Can you work these out from the model? Positions are in its coordinate system, mm. Coordinates: 2 decimals unless noted, no trailing zeros. Loops run counter-clockwise (first coordinate to the right, second up) from the corner with the lowest first, then second, coordinate; pieces in that order, holes last.
```python
from build123d import *

# Parameters (mm, degrees)
SKICA1_W                = 30
SKICA1_H                = 160
P_IDAT_VYSUNUT_M1_DEPTH = 10
ZAOBLIT1_R              = 10


with BuildPart() as part:
    # Skica1 → Přidat vysunutím1 (new body)
    with BuildSketch(Plane.XY):
        with Locations((15, 80)):
            Rectangle(SKICA1_W, SKICA1_H)
    extrude(amount=P_IDAT_VYSUNUT_M1_DEPTH)

    # Zaoblit1
    zaoblit1_edges = [part.edges().sort_by_distance(p)[0] for p in [
        (0, 160, 5),
        (30, 160, 5),
        (30, 0, 5),
        (0, 0, 5),
    ]]
    fillet(zaoblit1_edges, radius=ZAOBLIT1_R)


solid = part.part
```
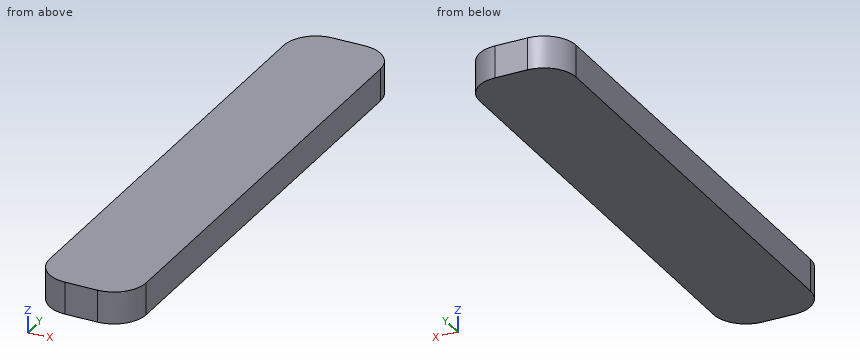
(1) I want a section at B-B on x = 2. Write out the boundary of the cut face in (y, z).
Check values:
outline: (4, 0) - (156, 0) - (156, 10) - (4, 10) - close
(2) I'm going to push a flat-ended pin straight in: pin 1 (6 mm diameter, centred on x = 26, z = 7.5, fed in from -Y). Where does the tip first touch, or does it pass through?
Check values:
pin 1: stops at y = 0.46
(3) If I drill on probe 1 along Y at (x, z) = (9.5, 9); probe 2 along Y at (x, z) = (23, 6); probe 3 along X at (y, z) = (151.5, 8.5), over which ranges is the centre line in solid material (lowest first)?
Check values:
probe 1: y = 0.01 to 159.99
probe 2: y = 0.46 to 159.54
probe 3: x = 0.11 to 29.89
(4) I want a section at A-A on z = 3. Write out the boundary of the cut face in (x, y).
Check values:
outline: (0, 10) arc R10 ccw to (10, 0) - (20, 0) arc R10 ccw to (30, 10) - (30, 150) arc R10 ccw to (20, 160) - (10, 160) arc R10 ccw to (0, 150) - close
(5) I want a section at C-C on x = 25.75. Write out the boundary of the cut face in (y, z).
Check values:
outline: (1.82, 0) - (158.18, 0) - (158.18, 10) - (1.82, 10) - close
